Geometry: final body of the model. Coordinates: model frame, mm. Face numbers are marked on the shaded views. A direction names the side the tool comes from. Coordinates: 2 decimals unless noted, no trailing zeros. Loops run counter-clockwise (first coordinate to the right, second up) from the corner with the lowest first, then second, coordinate; pieces in that order, holes last. Notation, with made-up numbers: (52.5, 50.25) - (58.5, 50.25) arc R28 ccw to (58.5, 82.25) - close; hole circle Ø10 at (76, 33.5). An arc over 180 degrees is marked (long way). Answer in a Markdown table with one row per item.
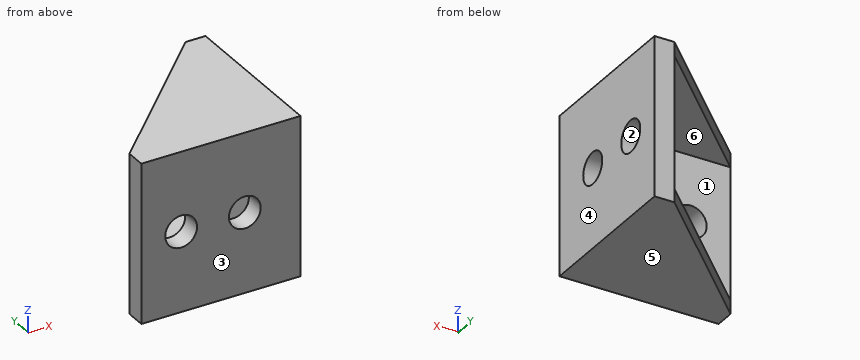
from build123d import *

# Parameters (mm, degrees)
EXTRUDE_1_DEPTH     = 20
CUT_EXTRUDE_START   = 20
SKETCH_2_W          = 17.5
SKETCH_2_H          = 16.6
CUT_EXTRUDE_1_DEPTH = 17.5
CUT_EXTRUDE_2_REACH = 36.641
SKETCH_3_R          = 2
CUT_EXTRUDE_3_REACH = 36.641
SKETCH_4_R          = 2


with BuildPart() as part:
    # 草图1 → 凸台-拉伸1 (new body)
    with BuildSketch(Plane.XY):
        Polygon((0, 0), (20, 0), (20, 20), (17.5, 20), (0, 2.5), align=None)
    extrude(amount=-EXTRUDE_1_DEPTH)

    # 草图2 → 切除-拉伸1 (cut)
    with BuildSketch(Plane(origin=(0, 0, 0), x_dir=(1, 0, 0), z_dir=(0, 1, 0)).offset(CUT_EXTRUDE_START)):
        with Locations((8.75, 10)):
            Rectangle(SKETCH_2_W, SKETCH_2_H)
    extrude(amount=-CUT_EXTRUDE_1_DEPTH, mode=Mode.SUBTRACT)

    # 草图3 → 切除-拉伸2 (cut, up to next)
    with BuildSketch(Plane(origin=(0, 0, 0), x_dir=(1, 0, 0), z_dir=(0, 1, 0)), mode=Mode.PRIVATE) as cut_extrude_2_sk1:
        with Locations(Location((5, 9.954039482, 0), (0, 0, 90))):
            Circle(SKETCH_3_R)
    cut_extrude_2_tool1 = extrude(cut_extrude_2_sk1.sketch, amount=CUT_EXTRUDE_2_REACH, mode=Mode.PRIVATE) & part.part
    # 草图3 → 切除-拉伸2 (cut, up to next)
    with BuildSketch(Plane(origin=(0, 0, 0), x_dir=(1, 0, 0), z_dir=(0, 1, 0)), mode=Mode.PRIVATE) as cut_extrude_2_sk2:
        with Locations(Location((13, 9.954039482, 0), (0, 0, 90))):
            Circle(SKETCH_3_R)
    cut_extrude_2_tool2 = extrude(cut_extrude_2_sk2.sketch, amount=CUT_EXTRUDE_2_REACH, mode=Mode.PRIVATE) & part.part
    add(cut_extrude_2_tool1.solids().sort_by_distance((5, 0, -9.954039))[0], mode=Mode.SUBTRACT)
    add(cut_extrude_2_tool2.solids().sort_by_distance((13, 0, -9.954039))[0], mode=Mode.SUBTRACT)

    # 草图4 → 切除-拉伸3 (cut, up to next)
    with BuildSketch(Plane(origin=(0, 0, 0), x_dir=(0, 0, -1), z_dir=(1, 0, 0)), mode=Mode.PRIVATE) as cut_extrude_3_sk1:
        with Locations(Location((10, 15, 0), (0, 0, 180))):
            Circle(SKETCH_4_R)
    cut_extrude_3_tool1 = extrude(cut_extrude_3_sk1.sketch, amount=CUT_EXTRUDE_3_REACH, mode=Mode.PRIVATE) & part.part
    # 草图4 → 切除-拉伸3 (cut, up to next)
    with BuildSketch(Plane(origin=(0, 0, 0), x_dir=(0, 0, -1), z_dir=(1, 0, 0)), mode=Mode.PRIVATE) as cut_extrude_3_sk2:
        with Locations(Location((10, 7, 0), (0, 0, 180))):
            Circle(SKETCH_4_R)
    cut_extrude_3_tool2 = extrude(cut_extrude_3_sk2.sketch, amount=CUT_EXTRUDE_3_REACH, mode=Mode.PRIVATE) & part.part
    add(cut_extrude_3_tool1.solids().sort_by_distance((0, 15, -10))[0], mode=Mode.SUBTRACT)
    add(cut_extrude_3_tool2.solids().sort_by_distance((0, 7, -10))[0], mode=Mode.SUBTRACT)


solid = part.part
(1) First-contact query: pin 1 Ø1 at (x, z) = (6, -14) entering from +Y; pin 2 Ø10 at (x, y) = (10, 14) entering from +Z; pin 3 Ø8.5 at (y, z) = (8, -8.5) entering from -X. Flat tips, straight axial feed; report the tip coordinate or a pass-through.
Verdict:
| item | result |
|---|---|
| pin 1 | stops at y = 2.5 |
| pin 2 | stops at z = 0 |
| pin 3 | stops at x = 17.5 |
(2) Cut plane A-A on y = 7. Output: boundary loops of the cut face in (x, z).
Verdict:
| item | result |
|---|---|
| outline | (4.5, -20) - (20, -20) - (20, -12) - (17.5, -12) - (17.5, -18.3) - (4.5, -18.3) - close; (4.5, -1.7) - (17.5, -1.7) - (17.5, -8) - (20, -8) - (20, 0) - (4.5, 0) - close |
(3) Cut plane D-D on z = -10. Output: boundary loops of the cut face in (x, y), then the cut area to 3 significant figures.
Verdict:
| item | result |
|---|---|
| outline | (0, 0) - (3, 0) - (3, 2.5) - (0, 2.5) - close; (7, 0) - (11, 0) - (11, 2.5) - (7, 2.5) - close; (15, 0) - (20, 0) - (20, 5) - (17.5, 5) - (17.5, 2.5) - (15, 2.5) - close; (17.5, 9) - (20, 9) - (20, 13) - (17.5, 13) - close; (17.5, 17) - (20, 17) - (20, 20) - (17.5, 20) - close |
| area | 53.8 mm² |
(4) Ray query, probe 1 along Y at (x, z) = (18.55, -10); probe 2 along Z at (x, y) = (13, 1.3); probe 3 along X at (y, z) = (2.25, -11). Return the intervals inside material, ascending.
Verdict:
| item | result |
|---|---|
| probe 1 | y = 0 to 5, 9 to 13, 17 to 20 |
| probe 2 | z = -20 to -11.95, -7.95 to 0 |
| probe 3 | x = 0 to 3.3, 6.7 to 11.3, 14.7 to 20 |
(5) Cut plane C-C on x = 10. Output: boundary loops of the cut face in (y, z), then the cut area to 3 significant figures.
Verdict:
| item | result |
|---|---|
| outline | (0, -20) - (12.5, -20) - (12.5, -18.3) - (2.5, -18.3) - (2.5, -1.7) - (12.5, -1.7) - (12.5, 0) - (0, 0) - close |
| area | 84.0 mm² |
(6) Access query for the marked faces 5 and 6. Directions: +Z, -Z, +X, -X, +Y, -Y. A direction counts if a zero-diameter tool reaches every point of the face in a straight line with its end or side. Return the directions, or none.
Verdict:
| item | result |
|---|---|
| face 5 | -Z, +X, -X, +Y, -Y |
| face 6 | -X, +Y |
(7) Cut plane B-B on x = 13. Output: boundary loops of the cut face in (y, z).
Verdict:
| item | result |
|---|---|
| outline | (0, -20) - (15.5, -20) - (15.5, -18.3) - (2.5, -18.3) - (2.5, -11.95) - (0, -11.95) - close; (0, -7.95) - (2.5, -7.95) - (2.5, -1.7) - (15.5, -1.7) - (15.5, 0) - (0, 0) - close |
(8) Pull-direction query (Y, two-part tool) for the marked faces 1, 2, 3 and 4; classes: pulls with the +Y half, pulls with the -Y half, needs draft (parallel to the pull), parting line crosses it, or undercut.
Verdict:
| item | result |
|---|---|
| face 1 | pulls with the +Y half |
| face 2 | undercut |
| face 3 | pulls with the -Y half |
| face 4 | needs draft |
